Autodesk Inventor part; units mm, degrees
ref_plane "YZ Plane" through (0, 0, 0) normal (1, 0, 0) x (0, 1, 0)
ref_plane "XZ Plane" through (0, 0, 0) normal (0, 1, 0) x (-1, 0, 0)
ref_plane "XY Plane" through (0, 0, 0) normal (0, 0, 1) x (1, 0, 0)
sketch "Sketch1" plane through (0, 0, 0) normal (0, 1, 0) x (-1, 0, 0)
  line L0 (-2.5, 7.5) -> (2.5, 7.5)
  line L1 (2.5, 7.5) -> (2.5, -7.5)
  line L2 (2.5, -7.5) -> (-2.5, -7.5)
  line L3 (-2.5, -7.5) -> (-2.5, 7.5)
  line L4 (-2.5, 7.5) -> (2.5, -7.5) construction
  line L5 (2.5, 7.5) -> (-2.5, -7.5) construction
  line L6 (-2.5, -7.5) -> (-9.5, -7.5)
  line L7 (-9.5, -7.5) -> (-9.5, 27.5)
  line L8 (-9.5, 27.5) -> (-2.5, 27.5)
  line L9 (-2.5, 27.5) -> (-2.5, -7.5)
  point P0 (0, 0)
  dimension "d0" = 5
  dimension "d1" = 15
  dimension "d13" = 35
  dimension "d14" = 7
extrude "Extrusion1" add sketch "Sketch1" along normal mid plane 3
sketch "Sketch3" plane through (0, -1.5, 0) normal (0, -1, 0) x (1, 0, 0)
  line L0 (1.1, 4.5) -> (-0.9, 4.5) construction
  line L1 (-0.9, 4.5) -> (-0.9, 2.5) construction
  line L2 (-0.9, 2.5) -> (1.1, 2.5) construction
  line L3 (1.1, 2.5) -> (1.1, 4.5) construction
  line L4 (1.1, 4.5) -> (-0.9, 2.5) construction
  line L5 (-0.9, 4.5) -> (1.1, 2.5) construction
  line L6 (1.1, -2.5) -> (-0.9, -2.5) construction
  line L7 (-0.9, -2.5) -> (-0.9, -4.5) construction
  line L8 (-0.9, -4.5) -> (1.1, -4.5) construction
  line L9 (1.1, -4.5) -> (1.1, -2.5) construction
  line L10 (1.1, -2.5) -> (-0.9, -4.5) construction
  line L11 (-0.9, -2.5) -> (1.1, -4.5) construction
  line L12 (0.1, 3.5) -> (0.1, -3.5) construction
  line L13 (-2.5, -7.5) -> (9.5, -7.5) construction
  line L14 (1.05, 2.55) -> (-0.85, 2.55)
  line L15 (-0.85, 2.55) -> (-0.85, 4.45)
  line L16 (-0.85, 4.45) -> (1.05, 4.45)
  line L17 (1.05, 4.45) -> (1.05, 2.55)
  line L18 (-0.85, -2.55) -> (1.05, -2.55)
  line L19 (1.05, -2.55) -> (1.05, -4.45)
  line L20 (1.05, -4.45) -> (-0.85, -4.45)
  line L21 (-0.85, -4.45) -> (-0.85, -2.55)
  line L22 (-2.5, 7.5) -> (-2.5, -7.5)
  point P0 (0, 0)
  point P1 (0.1, 0)
  dimension "d7" = 2
  dimension "d8" = 7
  dimension "d11" = 0.05
  dimension "d12" = 0.05
  dimension "d18" = 2.6
extrude "Extrusion3" add sketch "Sketch3" along normal blind 2
properties part number "RemovableAlignmentPiece"
Input: part model. Units: mm. Frame: model coordinates. A direction names the side the tool comes from. Round coordinates to 2 decimals unless told otherwise and drop trailing zeros. Loops run counter-clockwise (first coordinate to the right, second up) from the corner with the lowest first, then second, coordinate; pieces in that order, holes last. Notation, with made-up numbers: (15, 78.5) -> (44, 78.5) arc R32 cw to (44, 117.5) -> close; hole circle Ø9 at (45, 14.5). An arc over 180 degrees is marked (long way). One line per item, written item: value.
(1) Set-up query: faces 1 (the face through (0, -2, -2.55)), 2 (the face through (2.5, 0, 18)), 3 (the face through (1.05, -2, -3)). Return all of +Z, -Z, +X, -X, +Y, -Y with unobstructed straight access to the full face (end or side cutting, diameter ignored); none if empty.
Geometry check:
face 1: +X, -X, -Y
face 2: +Z, -X, +Y, -Y
face 3: +Z, -Z, +X, -Y
(2) Pin query (flat end, axial travel): pin 1 (2 mm diameter, centred on x = 4.5, y = -3, fed in from -Z); pin 2 (2 mm diameter, centred on x = 1.5, z = -1, fed in from -Y); pin 3 (0.6 mm diameter, centred on x = 0.5, y = -2.5, fed in from +Z); pin 4 (1 mm diameter, centred on y = -2.5, z = -3.5, fed in from +X). Return the tip coordinate at first contact, or that it passes through.
Geometry check:
pin 1: through
pin 2: y = -1.5
pin 3: z = 4.45
pin 4: x = 1.05
(3) Material intervals for line 1 (Z direction, x = -0.5, y = -2.6); line 2 (Y direction, x = 8.5, z = 1.5); line 3 (X direction, y = -1.1, z = 18), sorted ascending. Write a range as [from, to].
Geometry check:
line 1: [-4.45, -2.55], [2.55, 4.45]
line 2: [-1.5, 1.5]
line 3: [2.5, 9.5]
(4) Section A-A (y = -2.6). Return the cut outline in (x, z).
Geometry check:
outline: (-0.85, -4.45) -> (1.05, -4.45) -> (1.05, -2.55) -> (-0.85, -2.55) -> close; (-0.85, 2.55) -> (1.05, 2.55) -> (1.05, 4.45) -> (-0.85, 4.45) -> close
(5) Section B-B (z = 3.5). Return the cut outline in (x, y).
Geometry check:
outline: (-2.5, -1.5) -> (-0.85, -1.5) -> (-0.85, -3.5) -> (1.05, -3.5) -> (1.05, -1.5) -> (9.5, -1.5) -> (9.5, 1.5) -> (-2.5, 1.5) -> close
(6) Section C-C (x = 0.25). Return the cut outline in (y, z).
Geometry check:
outline: (-3.5, -4.45) -> (-1.5, -4.45) -> (-1.5, -7.5) -> (1.5, -7.5) -> (1.5, 7.5) -> (-1.5, 7.5) -> (-1.5, 4.45) -> (-3.5, 4.45) -> (-3.5, 2.55) -> (-1.5, 2.55) -> (-1.5, -2.55) -> (-3.5, -2.55) -> close
(7) Section D-D (y = 1.1). Return the cut outline in (x, z), plus the area to 3 significant figures.
Geometry check:
outline: (-2.5, -7.5) -> (9.5, -7.5) -> (9.5, 27.5) -> (2.5, 27.5) -> (2.5, 7.5) -> (-2.5, 7.5) -> close
area: 320 mm2
